Geometry: final body of the model. Coordinates: model frame, mm. A direction names the side the tool comes from. Round coordinates to 2 decimals unless told otherwise and drop trailing zeros. Loops run counter-clockwise (first coordinate to the right, second up) from the corner with the lowest first, then second, coordinate; pieces in that order, holes last. Notation, with made-up numbers: (79, -21) -> (117, -21) arc R35 cw to (117, 17) -> close; hole circle Ø11 at (52, 82). An arc over 180 degrees is marked (long way). Answer in a Markdown table with one row per item.
```python
from build123d import *

# Parameters (mm, degrees)
EXTRUDE_1_DEPTH     = 30
CUT_EXTRUDE_1_DEPTH = 45.676615807


with BuildPart() as part:
    # Эскиз1 → Вытянуть-Тонкостенный1 (new body)
    with BuildSketch(Plane.XY):
        Polygon((12, 0), (0, 0), (0, 30), (-2, 30), (-2, -2), (12, -2), align=None)
    extrude(amount=EXTRUDE_1_DEPTH)

    # Эскиз2 → Вытянуть1 (cut, through all)
    with BuildSketch(Plane.ZY.offset(2)):
        with BuildLine():
            Line((-0.098661396, 15.181132745), (-3.6788427, 15.181132745))
            Line((-3.6788427, 15.181132745), (-3.6788427, 31.57095784))
            Line((-3.6788427, 31.57095784), (33.600371965, 31.57095784))
            Line((33.600371965, 31.57095784), (33.600371965, 15.181132745))
            Line((33.600371965, 15.181132745), (30.098661396, 15.181132745))
            ThreePointArc((30.098661396, 15.181132745), (15, 29.966627674), (-0.098661396, 15.181132745))
        make_face()
    extrude(amount=-CUT_EXTRUDE_1_DEPTH, mode=Mode.SUBTRACT)


solid = part.part
```
Item 1: Pin query (flat end, axial travel): pin 1 Ø1 at (x, z) = (4, 15) entering from +Y; pin 2 Ø9 at (y, z) = (16.5, 11) entering from +X. Return the tip coordinate at first contact, or that it passes through.
Answer:
| item | result |
|---|---|
| pin 1 | stops at y = 0 |
| pin 2 | stops at x = 0 |
Item 2: Cut plane B-B (z = 10). Output: boundary loops of the cut face in (x, y), then the cut area to 3 significant figures.
Answer:
| item | result |
|---|---|
| outline | (-2, -2) -> (12, -2) -> (12, 0) -> (0, 0) -> (0, 29.11) -> (-2, 29.11) -> close |
| area | 86.2 mm² |
Item 3: Reachability of faces 1 (the face through (-0.2, 4.6, 0)), 2 (the face through (6, 0, 15)) from +Z, -Z, +X, -X, +Y, -Y: full face, straight path, thin tool, end or side. Return the list, or none.
Answer:
| item | result |
|---|---|
| face 1 | -Z, +X, -X, +Y, -Y |
| face 2 | +Z, -Z, +X, +Y |
Item 4: Line query: probe 1 along X at (y, z) = (20.5, 3.5); probe 2 along Z at (x, y) = (-0.5, 26). Output: solid intervals per line, ascending. Write a range as [from, to].
Answer:
| item | result |
|---|---|
| probe 1 | x = [-2, 0] |
| probe 2 | z = [4.8, 25.2] |
Item 5: Cut plane A-A (y = 0.5). Output: boundary loops of the cut face in (x, z), then the cut area to 3 significant figures.
Answer:
| item | result |
|---|---|
| outline | (-2, 0) -> (0, 0) -> (0, 30) -> (-2, 30) -> close |
| area | 60.0 mm² |
Item 6: Cut plane D-D (z = 13.5). Output: boundary loops of the cut face in (x, y), then the cut area to 3 significant figures.
Answer:
| item | result |
|---|---|
| outline | (-2, -2) -> (12, -2) -> (12, 0) -> (0, 0) -> (0, 29.89) -> (-2, 29.89) -> close |
| area | 87.8 mm² |
